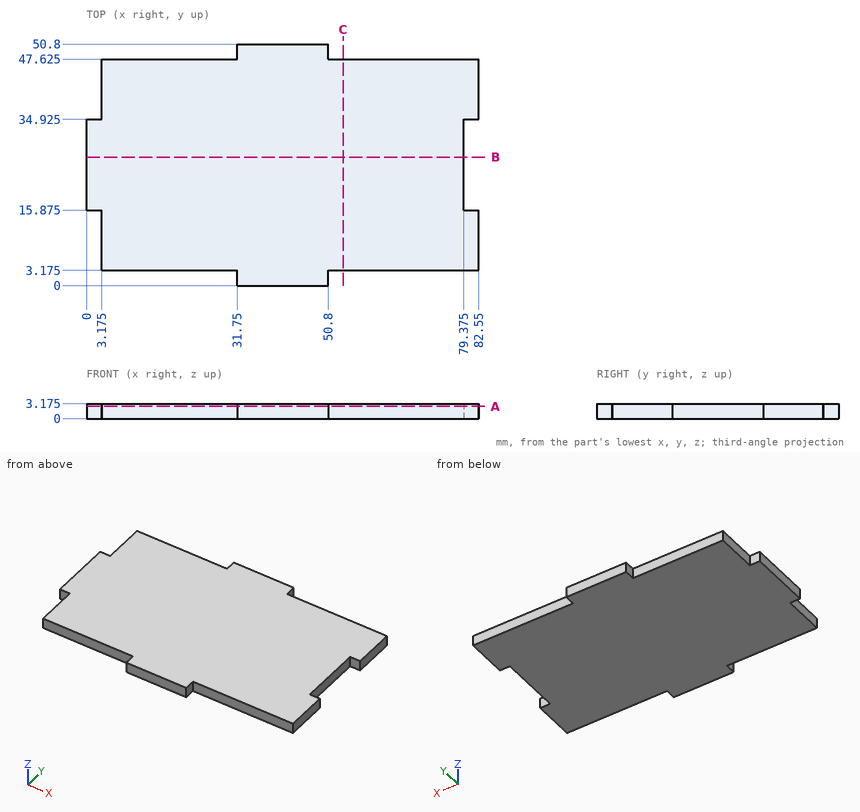
Source: three-view drawing plus pictorial views. Frame: mm from the lowest corner of the part. Round coordinates to 2 decimals unless told otherwise and drop trailing zeros. Order: outer loops, then holes, each group sorted by start corner. A loop starts at its lowest first (then second) coordinate and runs counter-clockwise, first axis right, second up. Notation, with made-up numbers: (-5.5, -23) -> (31.5, -23) arc R27 cw to (31.5, 3) -> close; hole circle Ø8 at (63, 66.5). An arc over 180 degrees is marked (long way). Use one line per item in the form item = value. Start each with the question number.
1. Line query: probe 1 along Y at (x, z) = (6, 2.4) (3 decimals); probe 2 along X at (y, z) = (6, 1.85) (3 decimals); probe 3 along X at (y, z) = (31, 2) (3 decimals). Output: solid intervals per line, ascending.
2. Cut plane A-A (z = 2.55). Return the cut outline in (x, y) (3 decimals), then the cut area to 3 significant figures.
3. Pin query (flat end, axial travel): pin 1 Ø1.6 at (x, z) = (1.5, 2) entering from +Y (3 decimals); pin 2 Ø1 at (x, z) = (81, 2) entering from -Y (3 decimals); pin 3 Ø1 at (y, z) = (1, 2) entering from -X. Return the tip coordinate at first contact, or that it passes through.
4. Cut plane C-C (x = 54). Return the cut outline in (y, z) (3 decimals).
5. Cut plane B-B (y = 27). Return the cut outline in (x, z) (3 decimals).
Solution:
q1.probe_1 = 3.175 to 47.625
q1.probe_2 = 3.175 to 82.55
q1.probe_3 = 0 to 79.375
q2.outline = (0, 15.875) -> (3.175, 15.875) -> (3.175, 3.175) -> (31.75, 3.175) -> (31.75, 0) -> (50.8, 0) -> (50.8, 3.175) -> (82.55, 3.175) -> (82.55, 15.875) -> (79.375, 15.875) -> (79.375, 34.925) -> (82.55, 34.925) -> (82.55, 47.625) -> (50.8, 47.625) -> (50.8, 50.8) -> (31.75, 50.8) -> (31.75, 47.625) -> (3.175, 47.625) -> (3.175, 34.925) -> (0, 34.925) -> close
q2.area = 3,650 mm^2
q3.pin_1 = 34.925
q3.pin_2 = 3.175
q3.pin_3 = 31.75
q4.outline = (3.175, 0) -> (47.625, 0) -> (47.625, 3.175) -> (3.175, 3.175) -> close
q5.outline = (0, 0) -> (79.375, 0) -> (79.375, 3.175) -> (0, 3.175) -> close
